Input: part model. Units: mm. Frame: model coordinates. A direction names the side the tool comes from. Give positions to 0.01 mm unless a question says otherwise; leave off trailing zeros. Write each loop counter-clockwise with the first axis right and the second up, starting at its lowest first coordinate (ties: lowest second). Pieces come first, ordered by that corner, then holes. Notation, with made-up numbers: (26.25, 34) - (51.25, 34) arc R9 cw to (51.25, 43) - close; hole circle Ø9 at (50, 73). An arc over 180 degrees is marked (long way). Use a Markdown table: item, result. Add a question column.
1. Section query A-A, the plane z = 33.5. Return loops of the section in (x, y), plus the area to 3 significant figures.
2. Pin query (flat end, axial travel): pin 1 (5 mm diameter, centred on x = 3, y = 14.5, fed in from -Z); pin 2 (2.5 mm diameter, centred on y = 3.5, z = 44, fed in from -X); pin 3 (3.5 mm diameter, centred on y = 22, z = 1, fed in from -X); pin 4 (4.5 mm diameter, centred on x = 2, y = 51, fed in from -Z). Return the tip coordinate at first contact, or that it passes through.
3. Section query D-D, the plane y = 5.6. Count the separate pieces of the cut face and the enclosed holes in it, plus the area to 3 significant figures.
4. Section query B-B, the plane x = 9. Return loops of the section in (y, z), plus the area to 3 significant figures.
5. Mould query, pull axis Z, two halves, no side actions, for faces 5 (the cylindrical face through (0.57, 7.9, 44.08)), 6 (the cylindrical face through (11.55, 50.9, 42.03)), 7 (the flat face through (11, 11, 37)). Classes: released by +Z, released by -Z, zero draft, split by the parting line, or undercut.
6. Material intervals for probe 1 along Z at (x, y) = (13.5, 26); probe 2 along Y at (x, z) = (2, 43.4); probe 3 along Y at (x, z) = (2.5, 2.1), sorted ascending.
7. Section query C-C, the plane z = 7. Return loops of the section in (x, y).
8. Set-up query: faces 1 (the cylindrical face through (0.6, 35.11, 1.52)), 2 (the cylindrical face through (2.934, 30.648, 45.107)), 3 (the flat face through (11, 19, 23)), 4 (the flat face through (9, 28, 42.6)). Return all of +Z, -Z, +X, -X, +Y, -Y with unobstructed straight access to the full face (end or side cutting, diameter ignored); none if empty.
```python
from build123d import *

# Parameters (mm, degrees)
BOSS_EXTRUDE1_DEPTH = 3
SKETCH2_R           = 1.35
SKETCH2_R_2         = 1.3
CUT_EXTRUDE1_DEPTH  = 59.051701095
SKETCH3_W           = 7
SKETCH3_H           = 4.5
BOSS_EXTRUDE2_DEPTH = 19.8
SKETCH4_W           = 4
SKETCH4_H           = 15
BOSS_EXTRUDE3_DEPTH = 19.8
SKETCH5_R           = 15
CUT_EXTRUDE2_DEPTH  = 2
SKETCH7_R           = 4.125
CUT_EXTRUDE3_DEPTH  = 0.5
SKETCH9_W           = 7.5
SKETCH9_H           = 15
BOSS_EXTRUDE4_DEPTH = 4.5
SKETCH12_R          = 1.35
CUT_EXTRUDE4_DEPTH  = 62.742125004
SKETCH13_W          = 3
SKETCH13_H          = 8
BOSS_EXTRUDE5_DEPTH = 1
FILLET1_R           = 2
SKETCH14_R          = 2
CUT_EXTRUDE5_DEPTH  = 1


with BuildPart() as part:
    # Sketch1 → Boss-Extrude1 (new body)
    with BuildSketch(Plane.XY):
        Polygon((0, 48), (6, 48), (6, 35.68), (0, 35.68), (0, 29.52), (6, 29.52), (6, 8.5), (0, 8.5), (0, 0), (15, 0), (15, 56), (0, 56), align=None)
    extrude(amount=BOSS_EXTRUDE1_DEPTH)

    # Sketch2 → Cut-Extrude1 (cut, through all)
    with BuildSketch(Plane.XY.offset(3)):
        with Locations((2, 51.5)):
            Circle(SKETCH2_R)
        with Locations((2.5, 5.6)):
            Circle(SKETCH2_R_2)
        with Locations((2.5, 32.6)):
            Circle(SKETCH2_R_2)
    extrude(amount=-CUT_EXTRUDE1_DEPTH, mode=Mode.SUBTRACT)

    # Sketch3 → Boss-Extrude2 (add)
    with BuildSketch(Plane.XY.offset(3)):
        with Locations((11.5, 53.75)):
            Rectangle(SKETCH3_W, SKETCH3_H)
    extrude(amount=BOSS_EXTRUDE2_DEPTH)

    # Sketch4 → Boss-Extrude3 (add)
    with BuildSketch(Plane.XY.offset(3)):
        with Locations((13, 11.5)):
            Rectangle(SKETCH4_W, SKETCH4_H)
    extrude(amount=BOSS_EXTRUDE3_DEPTH)

    # Sketch5 → Cut-Extrude2 (cut)
    with BuildSketch(Plane(origin=(15, 0, 0), x_dir=(0, 0, -1), z_dir=(1, 0, 0))):
        with Locations((-22.8, 12.56)):
            Circle(SKETCH5_R)
    extrude(amount=-CUT_EXTRUDE2_DEPTH, mode=Mode.SUBTRACT)

    # Sketch7 → Cut-Extrude3 (cut)
    with BuildSketch(Plane(origin=(13, 0, 0), x_dir=(0, 0, -1), z_dir=(1, 0, 0))):
        with Locations((-22.8, 12.56)):
            Circle(SKETCH7_R)
    extrude(amount=-CUT_EXTRUDE3_DEPTH, mode=Mode.SUBTRACT)

    # Sketch9 → Boss-Extrude4 (add)
    with BuildSketch(Plane.ZY.offset(-11)):
        with Locations((19.05, 11.5)):
            Rectangle(SKETCH9_W, SKETCH9_H)
    extrude(amount=BOSS_EXTRUDE4_DEPTH)

    # Sketch12 → Cut-Extrude4 (cut, through all)
    with BuildSketch(Plane(origin=(12.5, 0, 0), x_dir=(0, 0, -1), z_dir=(1, 0, 0))):
        with Locations((-22.8, 12.56)):
            Circle(SKETCH12_R)
    extrude(amount=-CUT_EXTRUDE4_DEPTH, mode=Mode.SUBTRACT)

    # Sketch13 → Boss-Extrude5 (add)
    with BuildSketch(Plane.ZY):
        with Locations((1.5, 52)):
            Rectangle(SKETCH13_W, SKETCH13_H)
    extrude(amount=BOSS_EXTRUDE5_DEPTH)

    # Fillet1
    fillet1_edges = [part.edges().sort_by_distance(p)[0] for p in [
        (6, 8.5, 1.5),
        (6, 29.52, 1.5),
        (6, 35.68, 1.5),
        (6, 48, 1.5),
        (11.5, 51.5, 3),
        (13, 19, 3),
        (13, 4, 3),
    ]]
    fillet(fillet1_edges, radius=FILLET1_R)
    fillet1_2_edges = [part.edges().sort_by_distance(p)[0] for p in [
        (-1, 56, 1.5),
        (-1, 48, 1.5),
        (0, 8.5, 1.5),
        (0, 29.52, 1.5),
        (0, 35.68, 1.5),
        (15, 56, 11.4),
        (0, 0, 1.5),
    ]]
    fillet(fillet1_2_edges, radius=FILLET1_R)

    # Mirror1: part across plane


with BuildPart() as part_1:
    add(part.part)
    add(part.part.mirror(Plane.XY.offset(22.8)))

    # Sketch14 → Cut-Extrude5 (cut)
    with BuildSketch(Plane(origin=(0, 0, 0), x_dir=(-1, 0, 0), z_dir=(0, 0, -1))):
        with Locations((-2, 51.5)):
            Circle(SKETCH14_R)
        with Locations((-2.5, 32.6)):
            Circle(SKETCH14_R)
        with Locations((-2.5, 5.6)):
            Circle(SKETCH14_R)
    cut_extrude5 = extrude(amount=-CUT_EXTRUDE5_DEPTH, mode=Mode.SUBTRACT)

    # Mirror2: Cut-Extrude5 across plane
    add(cut_extrude5.mirror(Plane(origin=(0, 0, 22.8), x_dir=(1, 0, 0), z_dir=(0, 0, -1))), mode=Mode.SUBTRACT)


solid = part_1.part
```
Result sheet:
| question | item | result |
|---|---|---|
| 1 | outline | (8, 51.5) - (15, 51.5) - (15, 54) arc R2 ccw to (13, 56) - (8, 56) - close; (11, 4) - (13, 4) - (13, 19) - (11, 19) - close |
| 1 | area | 60.6 mm² |
| 2 | pin 1 | passes through |
| 2 | pin 2 | stops at x = 0 |
| 2 | pin 3 | stops at x = 6 |
| 2 | pin 4 | stops at z = 0 |
| 3 | separate pieces | 3 |
| 3 | enclosed holes | 0 |
| 3 | area | 244 mm² |
| 4 | outline | (0, 0) - (56, 0) - (56, 45.6) - (0, 45.6) - (0, 42.6) - (49.5, 42.6) arc R2 cw to (51.5, 40.6) - (51.5, 5) arc R2 cw to (49.5, 3) - (0, 3) - close; (4, 15.3) - (19, 15.3) - (19, 30.3) - (4, 30.3) - close; hole circle Ø2.7 at (12.56, 22.8) |
| 4 | area | 735 mm² |
| 5 | face 5 | zero draft |
| 5 | face 6 | undercut |
| 5 | face 7 | undercut |
| 6 | probe 1 | z = 0 to 3, 42.6 to 45.6 |
| 6 | probe 2 | y = 0 to 4.4, 6.8 to 8.5, 29.52 to 31.4, 33.8 to 35.68, 48 to 50.15, 52.85 to 56 |
| 6 | probe 3 | y = 0 to 4.3, 6.9 to 8.5, 29.52 to 31.3, 33.9 to 35.68, 48 to 50.25, 52.75 to 56 |
| 7 | outline | (8, 51.5) - (15, 51.5) - (15, 54) arc R2 ccw to (13, 56) - (8, 56) - close; (11, 4) - (15, 4) - (15, 19) - (11, 19) - close |
| 8 | face 1 | +Z, -Z, -X |
| 8 | face 2 | +Z |
| 8 | face 3 | +X, -X |
| 8 | face 4 | -X |
